```python
from build123d import *

# Parameters (mm, degrees)
PAD_DEPTH       = 10
SKETCH002_R     = 5
PAD001_DEPTH    = 14
SKETCH003_R     = 4
PAD002_DEPTH    = 32
SKETCH004_R     = 5
PAD003_DEPTH    = 4
SKETCH005_R     = 4
PAD004_DEPTH    = 2
CHAMFER_SIZE    = 0.99
CHAMFER001_SIZE = 0.99
SKETCH006_R     = 5
PAD005_DEPTH    = 1
SKETCH007_R     = 4
PAD006_DEPTH    = 2
SKETCH008_R     = 5
PAD007_DEPTH    = 1
SKETCH009_R     = 4
PAD008_DEPTH    = 2
SKETCH010_R     = 5
PAD009_DEPTH    = 4
SKETCH011_R     = 6
PAD010_DEPTH    = 6
FILLET_R        = 0.99
FILLET001_R     = 1
SKETCH012_R     = 3.5
PAD011_DEPTH    = 10
CHAMFER002_SIZE = 0.99


with BuildPart() as part:
    # Sketch → Pad (new body)
    with BuildSketch(Plane.XY):
        with BuildLine():
            ThreePointArc((7.602809, 28.374071), (0, 29.375), (-7.602809, 28.374071))
            Line((-12.455667, 46.48518), (-7.602809, 28.374071))
            ThreePointArc((12.455667, 46.48518), (0, 48.125), (-12.455667, 46.48518))
            Line((7.602809, 28.374071), (12.455667, 46.48518))
        make_face()
    extrude(amount=PAD_DEPTH)

    # Sketch002 (on Face6 of Pad) → Pad001 (join)
    with BuildSketch(Plane.XY.offset(10)):
        with Locations((0, 38.75)):
            Circle(SKETCH002_R)
    extrude(amount=PAD001_DEPTH)

    # Sketch003 (on Face8 of Pad001) → Pad002 (join)
    with BuildSketch(Plane.XY.offset(24)):
        with Locations((0, 38.75)):
            Circle(SKETCH003_R)
    extrude(amount=PAD002_DEPTH)

    # Sketch004 (on Face10 of Pad002) → Pad003 (join)
    with BuildSketch(Plane.XY.offset(56)):
        with Locations((0, 38.75)):
            Circle(SKETCH004_R)
    extrude(amount=PAD003_DEPTH)

    # Sketch005 (on Face3 of Pad003) → Pad004 (join)
    with BuildSketch(Plane.XY.offset(60)):
        with Locations((0, 38.75)):
            Circle(SKETCH005_R)
    extrude(amount=PAD004_DEPTH)

    # Chamfer
    chamfer_edges = [part.edges().sort_by_distance(p)[0] for p in [
        (-4, 38.75, 24),
    ]]
    chamfer(chamfer_edges, length=CHAMFER_SIZE)

    # Chamfer001
    chamfer001_edges = [part.edges().sort_by_distance(p)[0] for p in [
        (-4, 38.75, 56),
    ]]
    chamfer(chamfer001_edges, length=CHAMFER001_SIZE)

    # Sketch006 (on Face15 of Chamfer001) → Pad005 (join)
    with BuildSketch(Plane.XY.offset(62)):
        with Locations((0, 38.75)):
            Circle(SKETCH006_R)
    extrude(amount=PAD005_DEPTH)

    # Sketch007 (on Face3 of Pad005) → Pad006 (join)
    with BuildSketch(Plane.XY.offset(63)):
        with Locations((0, 38.75)):
            Circle(SKETCH007_R)
    extrude(amount=PAD006_DEPTH)

    # Sketch008 (on Face7 of Pad006) → Pad007 (join)
    with BuildSketch(Plane.XY.offset(65)):
        with Locations((0, 38.75)):
            Circle(SKETCH008_R)
    extrude(amount=PAD007_DEPTH)

    # Sketch009 (on Face3 of Pad007) → Pad008 (join)
    with BuildSketch(Plane.XY.offset(66)):
        with Locations((0, 38.75)):
            Circle(SKETCH009_R)
    extrude(amount=PAD008_DEPTH)

    # Sketch010 (on Face7 of Pad008) → Pad009 (join)
    with BuildSketch(Plane.XY.offset(68)):
        with Locations((0, 38.75)):
            Circle(SKETCH010_R)
    extrude(amount=PAD009_DEPTH)

    # Sketch011 (on Face21 of Pad009) → Pad010 (join)
    with BuildSketch(Plane.XY.offset(10)):
        with Locations((0, 38.75)):
            Circle(SKETCH011_R)
    extrude(amount=PAD010_DEPTH)

    # Fillet
    fillet_edges = [part.edges().sort_by_distance(p)[0] for p in [
        (-6, 38.75, 16),
    ]]
    fillet(fillet_edges, radius=FILLET_R)

    # Fillet001
    fillet001_edges = [part.edges().sort_by_distance(p)[0] for p in [
        (-6, 38.75, 10),
    ]]
    fillet(fillet001_edges, radius=FILLET001_R)

    # Sketch012 (on Face30 of Fillet001) → Pad011 (join)
    with BuildSketch(Plane.XY.offset(72)):
        with Locations((0, 38.75)):
            Circle(SKETCH012_R)
    extrude(amount=PAD011_DEPTH)

    # Chamfer002
    chamfer002_edges = [part.edges().sort_by_distance(p)[0] for p in [
        (-4, 38.75, 68),
        (-4, 38.75, 65),
        (-4, 38.75, 62),
        (-4, 38.75, 66),
        (-4, 38.75, 63),
        (-4, 38.75, 60),
    ]]
    chamfer(chamfer002_edges, length=CHAMFER002_SIZE)


solid = part.part
```
Geometry check sheet. Reference: the model listing, model coordinates, mm. A direction names the side the tool comes from. Round coordinates to 2 decimals unless told otherwise and drop trailing zeros. Loops run counter-clockwise (first coordinate to the right, second up) from the corner with the lowest first, then second, coordinate; pieces in that order, holes last. Notation, with made-up numbers: (29, 77.25) - (61, 77.25) arc R13 ccw to (61, 93.25) - close; hole circle Ø8 at (22, 9.5). An arc over 180 degrees is marked (long way). Use a Markdown table: item, result.
Q1. Draft check along X on faces 1 (the flat face through (0, 39, 82)), 2 (the cylindrical face through (0.108, 29.375, 4.93)), 3 (the flat face through (-10.063, 37.556, 4.93)). Enter one of: released by +X, released by -X, zero draft, split by the parting line, or undercut.
Solutions:
| item | result |
|---|---|
| face 1 | zero draft |
| face 2 | undercut |
| face 3 | released by -X |
Q2. Cross-section at D-D on x = -10.25. Record the cut outline in (y, z).
Solutions:
| item | result |
|---|---|
| outline | (38.25, 0) - (47.02, 0) - (47.02, 10) - (38.25, 10) - close |
Q3. Material ranges on line 1 (Z direction, x = -1.75, y = 34.75); line 2 (Z direction, x = 2.25, y = 34.25); line 3 (X direction, y = 38.5, z = 14), recorded low to high.
Solutions:
| item | result |
|---|---|
| line 1 | z = 0 to 24.62, 55.38 to 60.62, 61.38 to 63.62, 64.38 to 66.62, 67.38 to 72 |
| line 2 | z = 0 to 16 |
| line 3 | x = -5.99 to 5.99 |
Q4. Go/stop test with flat-tipped pins: P1, Ø2, axis at x = 6.5, z = 24.5, coming from the -Y side; P2, Ø8, axis at y = 39, z = 67, coming from the -X side; P3, Ø5, axis at y = 38.5, z = 45, coming from the +X side; P4, Ø5, axis at x = -5.5, z = 40, coming from the -Y side. Record where each tip stops, or that it passes through.
Solutions:
| item | result |
|---|---|
| P1 | passes through |
| P2 | stops at x = -5 |
| P3 | stops at x = 4 |
| P4 | stops at y = 36.1 |
Q5. Access from +Z, -Z, +X, -X, +Y, -Y to the whole of each face (thin tool, end or side, straight path). Record for faces 4 (the flat face through (0, 38, 0)), 5 (the flat face through (-1.2, 42.2, 72)), 6 (the cylindrical face through (-0.521, 42.716, 39.79)).
Solutions:
| item | result |
|---|---|
| face 4 | -Z, +X, -X, +Y, -Y |
| face 5 | +Z |
| face 6 | none |
Q6. Cross-section at A-A on z = 76.5. Record the cut outline in (x, y).
Solutions:
| item | result |
|---|---|
| outline | circle Ø7 at (0, 38.75) |
Q7. Cross-section at B-B on x = 11.25. Record the cut outline in (y, z), plus the area to 3 significant figures.
Solutions:
| item | result |
|---|---|
| outline | (41.99, 0) - (46.79, 0) - (46.79, 10) - (41.99, 10) - close |
| area | 48.1 mm2 |
Q8. Cross-section at C-C on z = 32.5. Record the cut outline in (x, y), plus the area to 3 significant figures.
Solutions:
| item | result |
|---|---|
| outline | circle Ø8 at (0, 38.75) |
| area | 50.3 mm2 |
